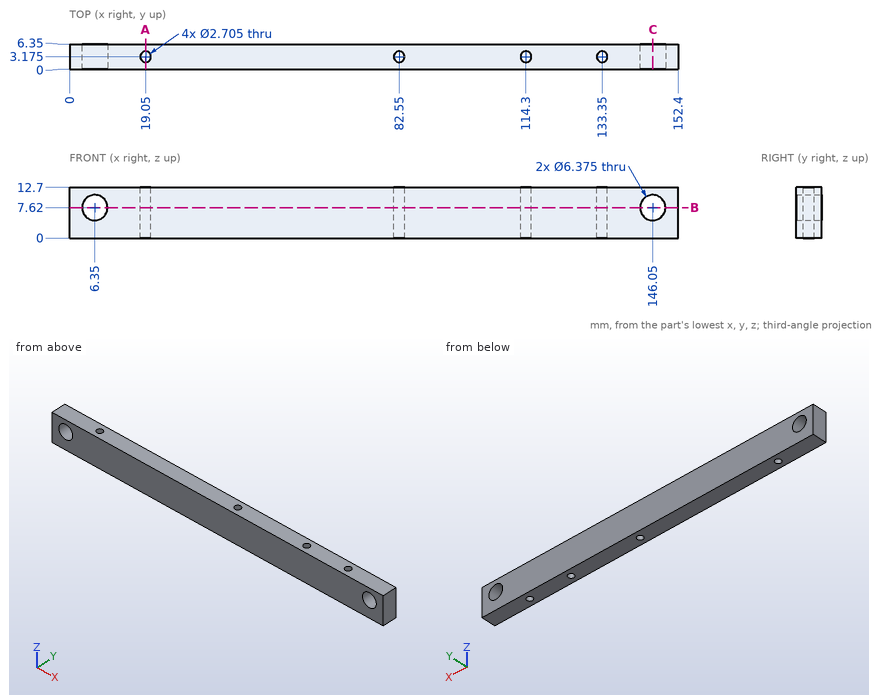
Answer from the drawing. Dimensions are ordinates in mm from the lowest x, y and z of the part. Give positions to 0.01 mm unless a question says otherwise; leave off trailing zeros. Write each loop counter-clockwise with the first axis right and the second up, starting at its lowest first coordinate (ties: lowest second). Pieces come first, ordered by that corner, then holes. Notation, with made-up numbers: (-38, -26) -> (-3, -26) arc R13 ccw to (-3, -18) -> close; hole circle Ø3 at (77.5, 74). An arc over 180 degrees is marked (long way). One line per question, with ' | ' between items. Start each with the question number.
1. Find the intervals of material crossed by probe 1 along Y at (x, z) = (82.55, 4.75); probe 2 along X at (y, z) = (4.25, 1.5); probe 3 along X at (y, z) = (5.5, 10.5) (1 decimal), in increasing order.
2. Section A-A (x = 19.05) is taken. Determine the outline of the cut face in (y, z).
3. Section C-C (x = 146.05) is taken. Determine the outline of the cut face in (y, z).
4. Section B-B (z = 7.62) is taken. State how many separate pieces and enclosed holes the cut face has.
5. Given pin 1 Ø2 at (x, y) = (19.05, 3.175) entering from +Z; pin 2 Ø3.5 at (x, y) = (133.35, 3.175) entering from -Z, each flat-ended and moving along its own axis, determine where each tip first touches the part or whether it passes through.
Response values:
1) probe 1: 0 to 1.82, 4.53 to 6.35 | probe 2: 0 to 18.23, 19.87 to 81.73, 83.37 to 113.48, 115.12 to 132.53, 134.17 to 152.4 | probe 3: 0 to 5, 7.7 to 144.7, 147.4 to 152.4
2) outline: (0, 0) -> (1.82, 0) -> (1.82, 12.7) -> (0, 12.7) -> close; (4.53, 0) -> (6.35, 0) -> (6.35, 12.7) -> (4.53, 12.7) -> close
3) outline: (0, 0) -> (6.35, 0) -> (6.35, 4.43) -> (0, 4.43) -> close; (0, 10.81) -> (6.35, 10.81) -> (6.35, 12.7) -> (0, 12.7) -> close
4) separate pieces: 3 | enclosed holes: 4
5) pin 1: through | pin 2: z = 0
